Read the model definition and answer for the solid it produces. Units are mm, in the model's axes. A direction names the side the tool comes from. Coordinates: 2 decimals unless noted, no trailing zeros. Write each loop counter-clockwise with the first axis right and the second up, starting at its lowest first coordinate (ties: lowest second). Pieces come first, ordered by that corner, then holes. Notation, with made-up numbers: (29, 50.5) - (82, 50.5) arc R20 cw to (82, 82.5) - close; hole circle Ø5 at (34, 36). An arc over 180 degrees is marked (long way). Return JSON: item names as keys, results as strings.
```python
from build123d import *

# Parameters (mm, degrees)
SKETCH1_W               = 80
SKETCH1_H               = 30
BOSS_EXTRUDE1_DEPTH     = 30
CUT_EXTRUDE1_DEPTH      = 91.553851381
CUT_EXTRUDE1_DEPTH_BACK = 91.553851381
SKETCH2_R               = 7.5
BOSS_EXTRUDE2_DEPTH     = 30
CUT_EXTRUDE2_DEPTH      = 109.453861158
CUT_EXTRUDE2_DEPTH_BACK = 109.453861158
SKETCH4_W               = 102.556598927
SKETCH4_H               = 19.243482925


with BuildPart() as part:
    # Sketch1 → Boss-Extrude1 (new body)
    with BuildSketch(Plane(origin=(0, 0, 0), x_dir=(1, 0, 0), z_dir=(0, 1, 0))):
        with Locations((40, 15)):
            Rectangle(SKETCH1_W, SKETCH1_H)
    extrude(amount=BOSS_EXTRUDE1_DEPTH)

    # Sketch2 → Cut-Extrude1 (cut, two sides: drawn at the far end of the back side and taken through both)
    with BuildSketch(Plane.XY.offset(-CUT_EXTRUDE1_DEPTH_BACK)):
        with Locations((61.5, 15)):
            Circle(SKETCH2_R)
        with Locations(Location((18.5, 15, 0), (0, 0, 180))):
            Circle(SKETCH2_R)
    extrude(amount=CUT_EXTRUDE1_DEPTH + CUT_EXTRUDE1_DEPTH_BACK, mode=Mode.SUBTRACT)

    # Sketch3 → Boss-Extrude2 (add)
    with BuildSketch(Plane.XY):
        Polygon((18.5, 30), (18.5, 59.856406461), (10.5, 30), align=None)
        Polygon((8.5, 66.8), (8.5, 61.8), (18.5, 61.8), (18.5, 59.856406461), (18.5, 30), (41.5, 30), (33.5, 59.856406461), (33.5, 66.8), align=None)
    extrude(amount=-BOSS_EXTRUDE2_DEPTH)

    # Sketch4 → Cut-Extrude2 (cut, two sides: drawn at the far end of the back side and taken through both)
    with BuildSketch(Plane.XY.offset(-CUT_EXTRUDE2_DEPTH_BACK)):
        with Locations((41.179129622, 5.378258538)):
            Rectangle(SKETCH4_W, SKETCH4_H)
    extrude(amount=CUT_EXTRUDE2_DEPTH + CUT_EXTRUDE2_DEPTH_BACK, mode=Mode.SUBTRACT)


solid = part.part
```
(1) A cutting plane is placed at A-A (z = -12.25). Determine the outline of the cut face in (x, y).
Answer:
{"outline": "(0, 15) - (11, 15) arc R7.5 cw to (26, 15) - (54, 15) arc R7.5 cw to (69, 15) - (80, 15) - (80, 30) - (41.5, 30) - (33.5, 59.86) - (33.5, 66.8) - (8.5, 66.8) - (8.5, 61.8) - (18.5, 61.8) - (18.5, 59.86) - (10.5, 30) - (0, 30) - close"}
(2) Straight lines are drawn through the part: line 1 (X direction, y = 20.5, z = -4.75); line 2 (Y direction, x = 7, z = -5.75); line 3 (X direction, y = 61.5, z = -8). For each, find the intervals that lie inside material, in ascending order. Write a range as from..to.
Answer:
{"line 1": "0..13.4, 23.6..56.4, 66.6..80", "line 2": "15..30", "line 3": "18.5..33.5"}
(3) A cutting plane is placed at B-B (x = 61.5). Determine the outline of the cut face in (y, z), and give its area (3 significant figures).
Answer:
{"outline": "(22.5, -30) - (30, -30) - (30, 0) - (22.5, 0) - close", "area": "225 mm²"}
(4) Flat-ended cylindrical pins translate along their axes: P1, Ø4, axis at y = 37.5, z = -4.5, coming from the -X side; P2, Ø9, axis at x = 56.5, z = -10.5, coming from the +Y side; P3, Ø2, axis at y = 60.5, z = -22.5, coming from the -X side. Find the tip coordinate at first contact, or state that the pin passes through.
Answer:
{"P1": "x = 11.97", "P2": "y = 30", "P3": "x = 18.4"}
(5) Which of the six approach directions +Z, -Z, +X, -X, +Y, -Y give full straight-line access (tool end or side, diameter ignored) to faces 1 (the face through (14.556, 45.137, -14.79)), 2 (the face through (60, 30, -15)), 3 (the face through (0, 22, -15))?
Answer:
{"face 1": "+Z, -Z, -X", "face 2": "+Z, -Z, +X, +Y", "face 3": "+Z, -Z, -X, +Y, -Y"}
(6) Determine the mould class of faces 4 (the face through (8.5, 64, -15)), 5 (the face through (5, 15, -15)), 6 (the face through (33.5, 63, -15)), 7 (the face through (18.66, 22.5, -15.21)) for opening direction X: +X half, -X half, draft (parallel to the pull), parting line (faces both ways), or undercut.
Answer:
{"face 4": "-X half", "face 5": "draft", "face 6": "+X half", "face 7": "undercut"}
(7) A cutting plane is placed at C-C (y = 63). Determine the outline of the cut face in (x, z), and give its area (3 significant figures).
Answer:
{"outline": "(8.5, -30) - (33.5, -30) - (33.5, 0) - (8.5, 0) - close", "area": "750 mm²"}
